Here's how the part is built. I have some questions about the finished solid (model axes, mm). A direction names the side the tool comes from. Round coordinates to 2 decimals unless told otherwise and drop trailing zeros. Write each loop counter-clockwise with the first axis right and the second up, starting at its lowest first coordinate (ties: lowest second). Pieces come first, ordered by that corner, then holes. Notation, with made-up numbers: (46.25, 35.5) - (92.25, 35.5) arc R12 ccw to (92.25, 46.5) - close; hole circle Ø3 at (63, -16.75). An arc over 180 degrees is marked (long way). Use one line per item in the form item = value. Start each with the question number.
1. I want a section at C-C, the plane z = 53. List the corners of the cut face in (x, y) for me, plus the area to 3 significant figures.
2. We'd pull the mould along Y, two halves only. Please class faces 1 (the flat face through (2, 0, 0)), 2 (the cylindrical face through (-1.5, -0.07, 51.77)), 3 (the flat face through (0, -2, 104)), 4 (the cylindrical face through (-1.08, -4.88, 51.33)): +Y half, -Y half, draft (parallel to the pull), parting line (faces both ways), or undercut.
3. Will these pins go through, and if not, where does the flat tip stop? pin 1 (2 mm diameter, centred on x = -0.5, z = 42, fed in from -Y); pin 2 (10 mm diameter, centred on y = 4.5, z = 23.5, fed in from +X); pin 3 (3 mm diameter, centred on x = -2, y = -1.5, fed in from +Z); pin 4 (1.5 mm diameter, centred on x = -0.5, y = -6.5, fed in from +Z).
4. Which directions (+Z, -Z, +X, -X, +Y, -Y) give clear straight access to the entire face, cutting with the end or side of a thin tool? Please do faces 5 (the cylindrical face through (-1.532, 3.695, 102.535)), 6 (the flat face through (0, 2, 105)).
5. If I drill on line 1 along Y through (x, z) = (0, 50); line 2 along Z through (x, y) = (5, 5.75), over which ranges is the centre line in solid material (lowest first)?
6. I want a section at A-A, the plane x = 0. List the corners of the cut face in (y, z) for me.
7. I want a section at B-B, the plane y = 0. List the corners of the cut face in (x, z) for me.
8. I want a section at D-D, the plane x = 7. List the corners of the cut face in (y, z) for me.
```python
from build123d import *

# Parameters (mm, degrees)
F0_R          = 8.5
F1_DEPTH      = 4
F3_R          = 5
F4_DEPTH      = 100
F5_W          = 4
F5_H          = 5
F9_DEPTH      = 8.501
F9_DEPTH_BACK = 25
F10_R         = 1.5
F11_DEPTH     = 110.8


with BuildPart() as f1:
    # F0 (on Top) → F1 (new body)
    with BuildSketch(Plane.XY):
        Circle(F0_R)
    extrude(amount=F1_DEPTH)

    # F3 (on Top) → F4 (join)
    with BuildSketch(Plane.XY):
        Circle(F3_R)
    extrude(amount=F4_DEPTH)

    # F5 (on Right) → F6 (revolve)
    with BuildSketch(Plane.YZ):
        with Locations((2, 102.5)):
            Rectangle(F5_W, F5_H)
    revolve(axis=Axis((0, 0, 102.5), (0, 0, -1)))

    # F8 (on Right) → F9 (cut, two sides)
    with BuildSketch(Plane.YZ) as f9_sk:
        Polygon((0, 106), (-5, 106), (-5, 101), align=None)
    extrude(amount=-F9_DEPTH, mode=Mode.SUBTRACT)
    extrude(f9_sk.sketch, amount=F9_DEPTH_BACK, mode=Mode.SUBTRACT)

    # F10 (on face) → F11 (cut)
    with BuildSketch(Plane(origin=(0, 0, 0), x_dir=(1, 0, 0), z_dir=(0, 0, -1))):
        Circle(F10_R)
    extrude(amount=-F11_DEPTH, mode=Mode.SUBTRACT)


solid = f1.part
```
Model answer:
q1.outline = circle Ø10 at (0, 0); hole circle Ø3 at (0, 0)
q1.area = 71.5 mm2
q2.face_1 = draft
q2.face_2 = undercut
q2.face_3 = -Y half
q2.face_4 = parting line
q3.pin_1 = -5
q3.pin_2 = 5
q3.pin_3 = 105
q3.pin_4 = 4
q4.face_5 = +Z
q4.face_6 = +Z, +X, -X, +Y, -Y
q5.line_1 = -5 to -1.5, 1.5 to 5
q5.line_2 = 0 to 4
q6.outline = (-8.5, 0) - (-1.5, 0) - (-1.5, 104.5) - (-4, 102) - (-4, 100) - (-5, 100) - (-5, 4) - (-8.5, 4) - close; (1.5, 0) - (8.5, 0) - (8.5, 4) - (5, 4) - (5, 100) - (4, 100) - (4, 105) - (1.5, 105) - close
q7.outline = (-8.5, 0) - (-1.5, 0) - (-1.5, 105) - (-4, 105) - (-4, 100) - (-5, 100) - (-5, 4) - (-8.5, 4) - close; (1.5, 0) - (8.5, 0) - (8.5, 4) - (5, 4) - (5, 100) - (4, 100) - (4, 105) - (1.5, 105) - close
q8.outline = (-4.82, 0) - (4.82, 0) - (4.82, 4) - (-4.82, 4) - close
